```python
from build123d import *

# Parameters (mm, degrees)
BOSS_EXTRUDE1_DEPTH = 8
SKETCH2_R           = 9
CUT_EXTRUDE1_DEPTH  = 35
SKETCH3_W           = 0.5
SKETCH3_H           = 1.875425002
CUT_EXTRUDE2_DEPTH  = 25
SKETCH4_R           = 2.5
CUT_EXTRUDE3_DEPTH  = 110
SKETCH6_W           = 5
SKETCH6_H           = 7.147198513
CUT_EXTRUDE4_DEPTH  = 10
FILLET1_R           = 0.5
SKETCH8_W           = 8
SKETCH8_H           = 3
BOSS_EXTRUDE2_DEPTH = 30
SKETCH9_R           = 9
CUT_EXTRUDE5_DEPTH  = 30
FILLET2_R           = 2
CUT_EXTRUDE7_DEPTH  = 30


with BuildPart() as part:
    # Sketch1 → Boss-Extrude1 (new body)
    with BuildSketch(Plane.XY):
        with BuildLine():
            Line((3.89007335, 2.5), (15, 2.5))
            Line((15, 2.5), (15, -2.5))
            Line((15, -2.5), (-15, -2.5))
            Line((-15, -2.5), (-15, 2.5))
            Line((-15, 2.5), (-3.89007335, 2.5))
            ThreePointArc((-3.89007335, 2.5), (0, 21.71234657), (3.89007335, 2.5))
        make_face()
    extrude(amount=BOSS_EXTRUDE1_DEPTH)

    # Sketch2 → Cut-Extrude1 (cut)
    with BuildSketch(Plane.XY.offset(8)):
        with Locations((0, 11.71234657)):
            Circle(SKETCH2_R)
    extrude(amount=-CUT_EXTRUDE1_DEPTH, mode=Mode.SUBTRACT)

    # Sketch3 → Cut-Extrude2 (cut)
    with BuildSketch(Plane(origin=(0, 0, 0), x_dir=(-1, 0, 0), z_dir=(0, 0, -1))):
        with Locations((0, 21.521483579)):
            Rectangle(SKETCH3_W, SKETCH3_H)
    extrude(amount=-CUT_EXTRUDE2_DEPTH, mode=Mode.SUBTRACT)

    # Sketch4 → Cut-Extrude3 (cut)
    with BuildSketch(Plane(origin=(15, 0, 0), x_dir=(0, 0, -1), z_dir=(1, 0, 0))):
        with Locations((-4, -2.5)):
            Circle(SKETCH4_R)
    extrude(amount=-CUT_EXTRUDE3_DEPTH, mode=Mode.SUBTRACT)

    # Sketch6 → Cut-Extrude4 (cut)
    with BuildSketch(Plane.XY.offset(8)):
        with Locations((0, 22.731746569)):
            Rectangle(SKETCH6_W, SKETCH6_H)
    extrude(amount=-CUT_EXTRUDE4_DEPTH, mode=Mode.SUBTRACT)

    # Fillet1
    fillet1_edges = [part.edges().sort_by_distance(p)[0] for p in [
        (-3.89007335, 2.5, 4),
        (3.89007335, 2.5, 4),
    ]]
    fillet(fillet1_edges, radius=FILLET1_R)

    # Sketch8 → Boss-Extrude2 (add)
    with BuildSketch(Plane.ZY.offset(15)):
        with Locations((4, 4)):
            Rectangle(SKETCH8_W, SKETCH8_H)
    extrude(amount=-BOSS_EXTRUDE2_DEPTH)

    # Sketch9 → Cut-Extrude5 (cut)
    with BuildSketch(Plane(origin=(0, 0, 0), x_dir=(-1, 0, 0), z_dir=(0, 0, -1))):
        with Locations((0, 11.71234657)):
            Circle(SKETCH9_R)
    extrude(amount=-CUT_EXTRUDE5_DEPTH, mode=Mode.SUBTRACT)

    # Fillet2
    fillet2_edges = [part.edges().sort_by_distance(p)[0] for p in [
        (-7.836245918, 5.5, 4),
        (7.836245918, 5.5, 4),
    ]]
    fillet(fillet2_edges, radius=FILLET2_R)

    # Sketch10 → Cut-Extrude7 (cut)
    with BuildSketch(Plane(origin=(0, 0, 0), x_dir=(-1, 0, 0), z_dir=(0, 0, -1))):
        with BuildLine():
            Line((0, 11.71234657), (3.420201433, 21.109272778))
            ThreePointArc((3.420201433, 21.109272778), (0, 24.529474212), (-3.420201433, 21.109272778))
            Line((-3.420201433, 21.109272778), (0, 11.71234657))
        make_face()
    extrude(amount=-CUT_EXTRUDE7_DEPTH, mode=Mode.SUBTRACT)


solid = part.part
```
Geometry check sheet. Reference: the model listing, model coordinates, mm. A direction names the side the tool comes from. Coordinates: 2 decimals unless noted, no trailing zeros. Order: outer loops, then holes, each group sorted by start corner. A loop starts at its lowest first (then second) coordinate and runs counter-clockwise, first axis right, second up.
Item 1: Scan lines: line 1 along X through (y, z) = (4.5, 4); line 2 along X through (y, z) = (5.75, 1.5); line 3 along Y through (x, z) = (-3.5, 4.25). Record each from-to range of solid material in increasing order.
Item 2: Section check C-C (z = 7). Enter the section's corners in (x, y), plus the area to 3 significant figures.
Item 3: Section check B-B (x = -5.5). Enter the section's corners in (y, z).
Item 4: Tool access check on faces 1 (the flat face through (13, 5.5, 4)), 2 (the flat face through (-13, 5.5, 4)), 3 (the flat face through (3.252, 20.646, 3.944)). Record the directions out of +Z, -Z, +X, -X, +Y, -Y that give a thin tool (end or side, any length) a straight path to the whole face; none if there is none.
Item 5: Depth check by flat-ended pin: pin 1 (1.9 mm diameter, centred on x = -14, z = 6, fed in from +Y); pin 2 (4 mm diameter, centred on x = -9.5, z = 3.5, fed in from +Y). Enter the tip coordinate at first touch or a pass-through.
Item 6: Mould release check, pull along X, two halves, no side actions. Record for faces 4 (the flat face through (1, 2, 8)), 5 (the flat face through (-15, 2, 4)), 6 (the flat face through (-3.247, 20.633, 3.944)): released by +X, released by -X, zero draft, split by the parting line, or undercut.
Item 7: Section check D-D (x = 0). Enter the section's corners in (y, z), plus the area to 3 significant figures.
Item 8: Section check A-A (y = 6.25). Enter the section's corners in (x, z).
Check sheet entries:
1. line 1: x = -15 to -5.38, 5.38 to 15
1. line 2: x = -10.27 to -6.74, 6.74 to 10.27
1. line 3: y = -0.01 to 3.42, 20 to 21.08
2. outline: (-15, -2.5) - (15, -2.5) - (15, 5.5) - (11.24, 5.5) arc R2 cw to (9.36, 8.2) arc R10 ccw to (3.42, 21.11) - (3.08, 20.17) arc R9 cw (long way) to (-3.08, 20.17) - (-3.42, 21.11) arc R10 ccw to (-9.36, 8.2) arc R2 cw to (-11.24, 5.5) - (-15, 5.5) - close
2. area: 256 mm2
3. outline: (-2.5, 0) - (4.59, 0) - (4.59, 8) - (-2.5, 8) - (-2.5, 6.5) arc R2.5 cw to (-2.5, 1.5) - close; (18.84, 0) - (20.06, 0) - (20.06, 8) - (18.84, 8) - close
4. face 1: +Z, -Z, +X, +Y
4. face 2: +Z, -Z, -X, +Y
4. face 3: +Z, -Z, +Y
5. pin 1: stops at y = 5.5
5. pin 2: stops at y = 18.33
6. face 4: zero draft
6. face 5: released by -X
6. face 6: undercut
7. outline: (-2.5, 0) - (2.71, 0) - (2.71, 8) - (-2.5, 8) - (-2.5, 6.5) arc R2.5 cw to (-2.5, 1.5) - close
7. area: 31.9 mm2
8. outline: (-9.68, 0) - (-7.15, 0) - (-7.15, 8) - (-9.68, 8) - close; (7.15, 0) - (9.68, 0) - (9.68, 8) - (7.15, 8) - close
